Can you work these out from the drawing? Everything is in mm from the part's minimum corner. Coordinates: 2 decimals unless noted, no trailing zeros. Order: outer loops, then holes, each group sorted by start corner. A loop starts at its lowest first (then second) coordinate and runs counter-clockwise, first axis right, second up. Notation, with made-up numbers: M -14,46 L 3,46 A18 cw 3,57 Z; hole C 68.5,-18.75 d1. An arc over 180 degrees is marked long. Answer as CSV lines item,"result". Start each with the question number.
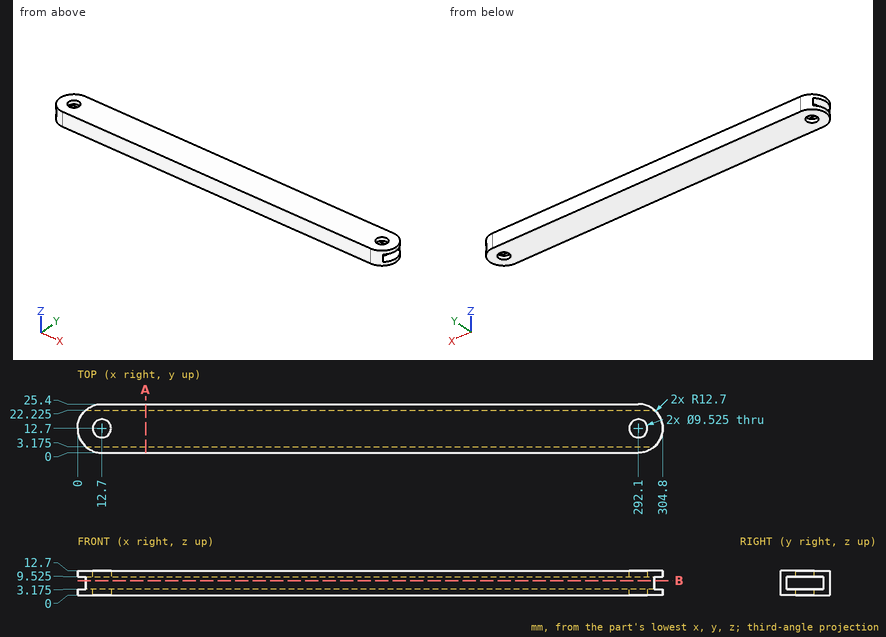
1) I need wall thicknesses on line 1 (Z direction, x = 172, y = 10) (3 decimals); line 2 (Y direction, x = 292, z = 10.75); line 3 (Y direction, x = 232, z = 7) (3 decimals). Which ranges of each line are inside material? Lowest first, please. Write a range as [from, to].
2) Suppose I cut it at A-A on x = 35.5. Please give me the cut outline in (y, z) (3 decimals), plus the area to 3 significant figures.
3) Will this pin go through, and if not, where does the flat tip stop? pin 1 Ø4 at (y, z) = (18.5, 3) entering from +X.
4) Suppose I cut it at B-B on z = 7.5. Please give me the cut outline in (x, y) (3 decimals).
Output:
1,line 1,"[0, 3.175], [9.525, 12.7]"
1,line 2,"[0, 7.94], [17.46, 25.4]"
1,line 3,"[0, 3.175], [22.225, 25.4]"
2,outline,"M 0,0 L 25.4,0 L 25.4,12.7 L 0,12.7 Z; hole M 3.175,3.175 L 22.225,3.175 L 22.225,9.525 L 3.175,9.525 Z"
2,area,"202 mm²"
3,pin 1,"x = 304.22"
4,outline,"M 4.3,3.175 A12.7 ccw 12.7,0 L 292.1,0 A12.7 ccw 300.5,3.175 Z; M 4.3,22.225 L 300.5,22.225 A12.7 ccw 292.1,25.4 L 12.7,25.4 A12.7 ccw Z"
